Work out the finished part from the listing and answer in its coordinate system (mm). A direction names the side the tool comes from. Coordinates: 2 decimals unless noted, no trailing zeros. Order: outer loops, then holes, each group sorted by start corner. A loop starts at its lowest first (then second) coordinate and runs counter-clockwise, first axis right, second up. Notation, with made-up numbers: M 0,74.25 L 21,74.25 A19 cw 21,99.25 Z; hole C 70.5,62.5 d9. An arc over 180 degrees is marked long. Use a Markdown table: item, result.
from build123d import *

# Parameters (mm, degrees)
SKETCH1_W          = 260
SKETCH1_H          = 160
TANK_BODY_DEPTH    = 300
INSIDE_START       = 297
SKETCH2_W          = 254
SKETCH2_H          = 154
INSIDE_DEPTH       = 294
INLET_PORT_START   = 300
SKETCH3_R          = 6
INLET_PORT_DEPTH   = 12
INLET_SOCKET_START = 312
SKETCH4_R          = 3.2
INLET_SOCKET_DEPTH = 10
INLET_HOLE_START   = 300
SKETCH5_R          = 2
INLET_HOLE_DEPTH   = 5
OUTLET_BOSS_START  = 80
SKETCH6_R          = 8
OUTLET_BOSS_DEPTH  = 6
TAP_SOCKET_START   = 86
SKETCH7_R          = 5.1
TAP_SOCKET_DEPTH   = 10


with BuildPart() as part:
    # Sketch1 → Tank_Body (new body)
    with BuildSketch(Plane(origin=(0, 0, 0), x_dir=(1, 0, 0), z_dir=(0, 1, 0))):
        Rectangle(SKETCH1_W, SKETCH1_H)
    extrude(amount=TANK_BODY_DEPTH)

    # Sketch2 → Inside (cut)
    with BuildSketch(Plane(origin=(0, 0, 0), x_dir=(1, 0, 0), z_dir=(0, 1, 0)).offset(INSIDE_START)):
        Rectangle(SKETCH2_W, SKETCH2_H)
    extrude(amount=-INSIDE_DEPTH, mode=Mode.SUBTRACT)

    # Sketch3 → Inlet_Port (add)
    with BuildSketch(Plane(origin=(0, 0, 0), x_dir=(1, 0, 0), z_dir=(0, 1, 0)).offset(INLET_PORT_START)):
        with Locations(Location((-105, 0, 0), (0, 0, 270))):
            Circle(SKETCH3_R)
    extrude(amount=INLET_PORT_DEPTH)

    # Sketch4 → Inlet_Socket (cut)
    with BuildSketch(Plane(origin=(0, 0, 0), x_dir=(1, 0, 0), z_dir=(0, 1, 0)).offset(INLET_SOCKET_START)):
        with Locations(Location((-105, 0, 0), (0, 0, 270))):
            Circle(SKETCH4_R)
    extrude(amount=-INLET_SOCKET_DEPTH, mode=Mode.SUBTRACT)

    # Sketch5 → Inlet_Hole (cut)
    with BuildSketch(Plane(origin=(0, 0, 0), x_dir=(1, 0, 0), z_dir=(0, 1, 0)).offset(INLET_HOLE_START)):
        with Locations(Location((-105, 0, 0), (0, 0, 270))):
            Circle(SKETCH5_R)
    extrude(amount=-INLET_HOLE_DEPTH, mode=Mode.SUBTRACT)

    # Sketch6 → Outlet_Boss (add)
    with BuildSketch(Plane.XY.offset(OUTLET_BOSS_START)):
        with Locations((0, 60)):
            Circle(SKETCH6_R)
    extrude(amount=OUTLET_BOSS_DEPTH)

    # Sketch7 → Tap_Socket (cut)
    with BuildSketch(Plane.XY.offset(TAP_SOCKET_START)):
        with Locations((0, 60)):
            Circle(SKETCH7_R)
    extrude(amount=-TAP_SOCKET_DEPTH, mode=Mode.SUBTRACT)


solid = part.part
1. Flat-ended cylindrical pins translate along their axes: P1, Ø2, axis at x = 86, z = 53, coming from the +Y side; P2, Ø1.9, axis at x = -104, z = -1, coming from the +Y side; P3, Ø5, axis at x = 15, y = 150, coming from the +Z side. Find the tip coordinate at first contact, or state that the pin passes through.
Answers below:
| item | result |
|---|---|
| P1 | y = 300 |
| P2 | y = 302 |
| P3 | z = 80 |
2. Find the intervals of material crossed by probe 1 along Y at (x, z) = (-91, -31.5); probe 2 along Z at (x, y) = (54, 289); probe 3 along X at (y, z) = (155, -23), in increasing order.
Answers below:
| item | result |
|---|---|
| probe 1 | 0 to 3, 297 to 300 |
| probe 2 | -80 to -77, 77 to 80 |
| probe 3 | -130 to -127, 127 to 130 |
3. Section A-A on x = 14.5 is taken. Determine the outline of the cut face in (y, z).
Answers below:
| item | result |
|---|---|
| outline | M 0,-80 L 300,-80 L 300,80 L 0,80 Z; hole M 3,-77 L 297,-77 L 297,77 L 3,77 Z |
4. Section C-C on y = 60 is taken. Determine the outline of the cut face in (x, z), then the cut area to 3 significant figures.
Answers below:
| item | result |
|---|---|
| outline | M -130,-80 L 130,-80 L 130,80 L 8,80 L 8,86 L 5.1,86 L 5.1,77 L 127,77 L 127,-77 L -127,-77 L -127,77 L -5.1,77 L -5.1,86 L -8,86 L -8,80 L -130,80 Z |
| area | 2,490 mm² |
5. For a pull along Z with two mould halves and no side action, classify faces 4 (the face through (-127, 152, 1)), 5 (the face through (-99.05, 305.92, -0.78)), 6 (the face through (5, 58, 86)) as +Z half, -Z half, draft (parallel to the pull), parting line (faces both ways), or undercut.
Answers below:
| item | result |
|---|---|
| face 4 | undercut |
| face 5 | parting line |
| face 6 | +Z half |
6. For faces 1 (the face through (-1, 65, 82)), 2 (the face through (-2, 152, -77)), 3 (the face through (-108, 312, 3)), determine the directions among +Z, -Z, +X, -X, +Y, -Y from which every point of the face is accessible in a straight line to the end or side of a thin tool.
Answers below:
| item | result |
|---|---|
| face 1 | +Z |
| face 2 | none |
| face 3 | +Z, -Z, +X, -X, +Y |
7. Section B-B on y = 177 is taken. Determine the outline of the cut face in (x, z).
Answers below:
| item | result |
|---|---|
| outline | M -130,-80 L 130,-80 L 130,80 L -130,80 Z; hole M -127,-77 L 127,-77 L 127,77 L -127,77 Z |
